For this review, take the finished solid that the model builds, in its own axes (mm). A direction names the side the tool comes from. Round coordinates to 2 decimals unless told otherwise and drop trailing zeros. Order: outer loops, then holes, each group sorted by start corner. A loop starts at its lowest first (then second) coordinate and runs counter-clockwise, first axis right, second up. Notation, with made-up numbers: M 73.25,89.25 L 80.25,89.25 A9 cw 80.25,94.25 Z; hole C -3,29.25 d5. An arc over 180 degrees is marked long. Put each result on its own line as item: value.
from build123d import *

# Parameters (mm, degrees)
SKETCH001_W     = 7
SKETCH001_H     = 7
PAD001_DEPTH    = 8.5
POCKET_DEPTH    = 7
SKETCH003_R     = 1.4
POCKET001_DEPTH = 5
SKETCH004_W     = 2.8
SKETCH004_H     = 3.5
POCKET002_DEPTH = 4


with BuildPart() as part:
    # Sketch001 (on Face1 of CopyFillet) → Pad001 (new body)
    with BuildSketch(Plane.XY.offset(1.6)):
        with Locations((0, 8.999962)):
            Rectangle(SKETCH001_W, SKETCH001_H)
    extrude(amount=PAD001_DEPTH)

    # Sketch002 (on Face2 of Pad001) → Pocket (cut)
    with BuildSketch(Plane(origin=(3.5, 0, 1.6), x_dir=(0, 1, 0), z_dir=(1, 0, 0))):
        Polygon((5.499962, 4.5), (6.749962, 8.5), (5.499962, 8.5), align=None)
        Polygon((11.249962, 8.5), (12.499962, 8.5), (12.499962, 4.5), align=None)
    extrude(amount=-POCKET_DEPTH, mode=Mode.SUBTRACT)

    # Sketch003 (on Face8 of Pocket) → Pocket001 (cut)
    with BuildSketch(Plane.XY.offset(10.1)):
        with Locations((-1.75, 8.999962)):
            Circle(SKETCH003_R)
        with Locations((1.75, 8.999962)):
            Circle(SKETCH003_R)
    extrude(amount=-POCKET001_DEPTH, mode=Mode.SUBTRACT)

    # Sketch004 (on Face6 of Pocket001) → Pocket002 (cut)
    with BuildSketch(Plane(origin=(0, 12.499962, 1.6), x_dir=(-1, 0, 0), z_dir=(0, 1, 0))):
        with Locations((-1.75, 2.25)):
            Rectangle(SKETCH004_W, SKETCH004_H)
        with Locations((1.75, 2.25)):
            Rectangle(SKETCH004_W, SKETCH004_H)
    extrude(amount=-POCKET002_DEPTH, mode=Mode.SUBTRACT)


solid = part.part
(1) Add section C-C on z = 2.5. Give the boundary of the cut face in (x, y).
A:
outline: M -3.5,5.5 L 3.5,5.5 L 3.5,12.5 L 3.15,12.5 L 3.15,8.5 L 0.35,8.5 L 0.35,12.5 L -0.35,12.5 L -0.35,8.5 L -3.15,8.5 L -3.15,12.5 L -3.5,12.5 Z
(2) For faces 4 (the face through (2, 8, 5.1)), 5 (the face through (0, 9, 10.1)), 6 (the face through (0.049, 6.116, 8.072)), 7 (the face through (-2.053, 7.633, 7.635)), 8 (the face through (2, 11, 2.1)), list the 3-axis set-ups (+Z, -Z, +X, -X, +Y, -Y) from which the entire face can be reached by the end or side of a thin tool; tool diameter is ignored.
A:
face 4: +Z, +Y
face 5: +Z, +X, -X, +Y, -Y
face 6: +Z, +X, -X, -Y
face 7: +Z
face 8: +Y
(3) To check wall thickness, follow L1, parallel to X at y = 9.5, z = 3.75; L2, parallel to Y at x = -2.75, z = 4.75. State the ranges of each line that lie inside material, in increasing order.
A:
L1: x = -3.5 to -3.15, -0.35 to 0.35, 3.15 to 3.5
L2: y = 5.5 to 8.5
(4) Add section B-B on x = -1.75. Give the boundary of the cut face in (y, z), then the cut area to 4 significant figures.
A:
outline: M 5.5,1.6 L 12.5,1.6 L 12.5,2.1 L 8.5,2.1 L 8.5,5.1 L 7.6,5.1 L 7.6,10.1 L 6.75,10.1 L 5.5,6.1 Z; M 10.4,5.6 L 12.5,5.6 L 12.5,6.1 L 11.25,10.1 L 10.4,10.1 Z
area: 27.45 mm2
(5) Insertion check: pin 1 Ø0.8 at (x, z) = (-2, 3.5) entering from +Y; pin 2 Ø0.5 at (x, y) = (2, 8) entering from +Z. Each pin has a flat end and moves straight along its axis. Give the tip position at first contact, or say it passes through.
A:
pin 1: stops at y = 8.5
pin 2: stops at z = 5.1
(6) Draft analysis for pull direction X (two halves, no side actions). For faces 1 (the face through (-2, 8.5, 3)), 2 (the face through (3.5, 9, 6)), 3 (the face through (0.049, 11.884, 8.072)), state which applies: released by +X, released by -X, zero draft, split by the parting line, or undercut.
A:
face 1: undercut
face 2: released by +X
face 3: zero draft
(7) Add section A-A on y = 11. Give the boundary of the cut face in (x, z).
A:
outline: M -3.5,1.6 L 3.5,1.6 L 3.5,10.1 L -3.5,10.1 Z; hole M -3.15,2.1 L -0.35,2.1 L -0.35,5.6 L -3.15,5.6 Z; hole M 0.35,2.1 L 3.15,2.1 L 3.15,5.6 L 0.35,5.6 Z
(8) Add section D-D on y = 8.25. Give the boundary of the cut face in (x, z), then the cut area to 3 significant figures.
A:
outline: M -3.5,1.6 L 3.5,1.6 L 3.5,10.1 L 2.93,10.1 L 2.93,5.1 L 0.57,5.1 L 0.57,10.1 L -0.57,10.1 L -0.57,5.1 L -2.93,5.1 L -2.93,10.1 L -3.5,10.1 Z
area: 35.9 mm2
